Solid Edge part; units mm, degrees
sketch "Sketch1" plane through (0, 0, 0) normal (0, 0, 1) x (1, 0, 0)
  line L0 (4, 20) -> (4, -20)
  line L1 (-4, 20) -> (-4, -20)
  arc A0 (4, -20) -> (-4, -20) centre (0, -20) cw
  arc A1 (-4, 20) -> (4, 20) centre (0, 20) cw
  circle A2 centre (0, -20) radius 1.5
  circle A3 centre (0, 20) radius 1.5
extrude "Protrusion1" add sketch "Sketch1" along normal blind 8
sketch "Sketch2" plane through (4, 0, 4) normal (1, 0, 0) x (0, 1, 0)
  line L0 (16, 2) -> (-16, 2)
  line L1 (-16, 2) -> (-16, -2)
  line L2 (-16, -2) -> (16, -2)
  line L3 (16, -2) -> (16, 2)
extrude "VaciadoExtruido_1" cut sketch "Sketch2" against normal blind 2
chamfer "Chaflán_1" distance 2 angle 45 4 edges at (2, 0, 2) (2, 16, 4) (2, 0, 6) (2, -16, 4)
mirror "Mirror1" about plane through (0, 0, 0) normal (1, 0, 0) of "VaciadoExtruido_1"
chamfer "Chamfer1" distance 2 angle 45 4 edges at (-2, 0, 2) (-2, 16, 4) (-2, 0, 6) (-2, -16, 4)
chamfer "Chaflán_3" distance 0.5 angle 45 10 edges at (-4, 0, 8) (0, 24, 8) (4, 0, 8) (-4, 0, 0) (0, 24, 0) (4, 0, 0) (-1.5, -20, 8) (-1.5, 20, 8) (-1.5, 20, 0) (-1.5, -20, 0)
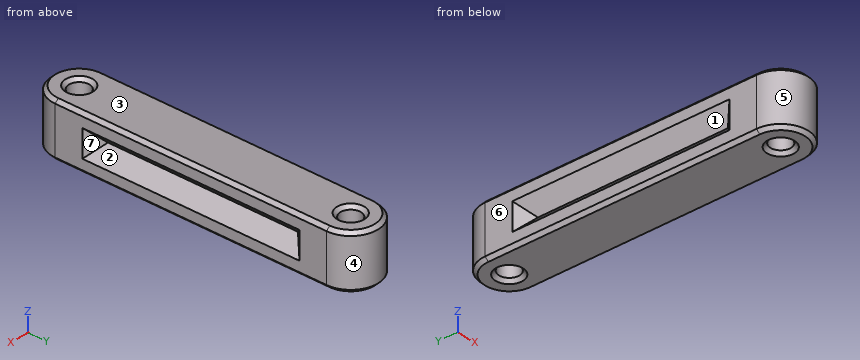
Verification items for the finished model (mm, model axes). Face numbers are marked on the shaded views. A direction names the side the tool comes from. Give positions to 0.01 mm unless a question says otherwise; leave off trailing zeros. Write each loop counter-clockwise with the first axis right and the second up, starting at its lowest first coordinate (ties: lowest second). Pieces come first, ordered by that corner, then holes. Notation, with made-up numbers: (-13.75, 16.25) - (1.25, 16.25) arc R20 ccw to (1.25, 20.25) - close; hole circle Ø7 at (12.5, -26.75). An arc over 180 degrees is marked (long way). Answer as CSV lines item,"result". Start each with the question number.
1. Sectioned sample at A-A (x = 0). Record the boundary of the cut face in (y, z), then the cut area to 4 significant figures.
2. Thickness scan on line 1 (Y direction, x = 0, z = 5.5); line 2 (Y direction, x = 1, z = 1.75); line 3 (Z direction, x = -2.75, y = 9). Record the ranges inside material, lowest first.
3. Set-up check for the marked faces 1, 2 and 3: record each of +Z, -Z, +X, -X, +Y, -Y from which the full face is reachable in a straight line by a thin tool's end or side.
4. Depth check by flat-ended pin: pin 1 (2 mm diameter, centred on x = 1.5, z = 2, fed in from +Y). Enter the tip coordinate at first touch or a pass-through.
5. Draft check along Y on the marked faces 4, 5, 6 and 7. Enter one of: pulls with the +Y half, pulls with the -Y half, needs draft (parallel to the pull), parting line crosses it, or undercut.
6. Sectioned sample at C-C (z = 5). Count the separate pieces of the cut face and the enclosed holes in it, then the cut area to 3 significant figures.
Derived:
1,outline,"(-24, 0.5) - (-23.5, 0) - (-22, 0) - (-21.5, 0.5) - (-21.5, 7.5) - (-22, 8) - (-23.5, 8) - (-24, 7.5) - close; (-18.5, 0.5) - (-18, 0) - (18, 0) - (18.5, 0.5) - (18.5, 7.5) - (18, 8) - (-18, 8) - (-18.5, 7.5) - close; (21.5, 0.5) - (22, 0) - (23.5, 0) - (24, 0.5) - (24, 7.5) - (23.5, 8) - (22, 8) - (21.5, 7.5) - close"
1,area,"334.5 mm²"
2,line 1,"-24 to -21.5, -18.5 to 18.5, 21.5 to 24"
2,line 2,"-23.87 to -21.12, -18.88 to 18.88, 21.12 to 23.87"
2,line 3,"0 to 3.25, 4.75 to 8"
3,face 1,"-X"
3,face 2,"+X"
3,face 3,"+Z, +X, -X, +Y, -Y"
4,pin 1,"y = 23.97"
5,face 4,"pulls with the +Y half"
5,face 5,"pulls with the -Y half"
5,face 6,"needs draft"
5,face 7,"undercut"
6,separate pieces,"1"
6,enclosed holes,"2"
6,area,"294 mm²"
